Can you work these out from the model? Positions are in its coordinate system, mm. Face numbers are marked on the shaded views. Round coordinates to 2 decimals unless told otherwise and drop trailing zeros. Loops run counter-clockwise (first coordinate to the right, second up) from the corner with the lowest first, then second, coordinate; pieces in that order, holes last. Notation, with made-up numbers: (44.5, 27.5) -> (91.5, 27.5) arc R24 cw to (91.5, 44.5) -> close; hole circle Ø4 at (22, -34.5). An arc over 180 degrees is marked (long way). Write each question's results on one line, items separated by ' | '.
from build123d import *

# Parameters (mm, degrees)
SKETCH1_W           = 1270
SKETCH1_H           = 1016
SKETCH1_W_2         = 254
BOSS_EXTRUDE1_DEPTH = 1016


with BuildPart() as part:
    # Sketch1 → Boss-Extrude1 (new body)
    with BuildSketch(Plane.XY):
        with Locations((889, 508)):
            Rectangle(SKETCH1_W, SKETCH1_H)
        with Locations((127, 508)):
            Rectangle(SKETCH1_W_2, SKETCH1_H)
    extrude(amount=BOSS_EXTRUDE1_DEPTH)

    # SurfaceCut2
    split(bisect_by=Plane(origin=(555.355932203, 925.593220339, 925.593220339), x_dir=(-0.9205746178983233, 0.27617238536949706, 0.27617238536949706), z_dir=(-0.3905667329424717, -0.6509445549041193, -0.6509445549041194)), keep=Keep.TOP)

    # SurfaceCut3
    split(bisect_by=Plane(origin=(297.050847458, -495.084745763, 495.084745763), x_dir=(-0.9205746178983234, -0.27617238536949706, 0.2761723853694971), z_dir=(-0.39056673294247174, 0.6509445549041194, -0.6509445549041194)), keep=Keep.TOP)

    # SurfaceCut4
    split(bisect_by=Plane(origin=(205.153846154, 0, 1025.769230769), x_dir=(-0.9805806756909202, 0, 0.196116135138184), z_dir=(-0.196116135138184, 0, -0.9805806756909202)), keep=Keep.TOP)


solid = part.part
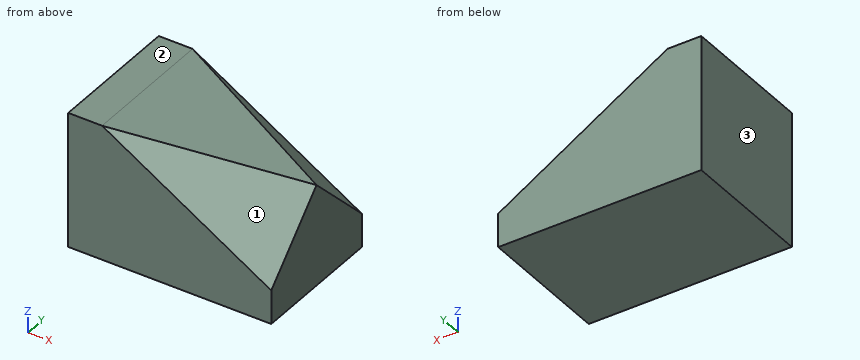
1. We'd pull the mould along X, two halves only. Please class the marked faces 1, 2 and 3: pulls with the +X half, pulls with the -X half, needs draft (parallel to the pull), parting line crosses it, or undercut.
Final values:
face 1: pulls with the +X half | face 2: needs draft | face 3: pulls with the -X half
2. Will these pins go through, and if not, where does the flat tip stop? pin 1 (2 mm diameter, centred on x = 391.5, z = 656, fed in from -Y); pin 2 (2 mm diameter, centred on y = 191, z = 606.5, fed in from +X); pin 3 (1.5 mm diameter, centred on x = 750.5, y = 551, fed in from +Z); pin 4 (8 mm diameter, centred on x = 1245, y = 186.5, fed in from +Z).
Final values:
pin 1: y = 0 | pin 2: x = 1257.19 | pin 3: z = 916.85 | pin 4: z = 612.56
3. If we section it at A-A (z = 708.5): List the corners of the cut face in (x, y) for me.
Final values:
outline: (0, 0) -> (766.5, 0) -> (1524, 454.5) -> (1524, 561.5) -> (766.5, 1016) -> (0, 1016) -> close
4. Please list where these lines run through material, in increasing order: line 1 (Z direction, x = 814.5, y = 884); line 2 (Z direction, x = 1406, y = 631); line 3 (X direction, y = 61, z = 602.5). Write a range as from..to.
Final values:
line 1: 0..811.7 | line 2: 0..709.8 | line 3: 0..1044.83
5. If we section it at B-B (x = 615.5): List the corners of the cut face in (y, z) for me, then the cut area to 3 significant figures.
Final values:
outline: (0, 0) -> (1016, 0) -> (1016, 799.1) -> (871.4, 943.7) -> (144.6, 943.7) -> (0, 799.1) -> close | area: 938,000 mm2
